```python
from build123d import *

# Parameters (mm, degrees)
SKETCH_1_R          = 13
EXTRUDE_1_DEPTH     = 5
SKETCH_2_R          = 12
CUT_EXTRUDE_1_DEPTH = 3
SKETCH_3_R          = 2.5
CUT_EXTRUDE_2_DEPTH = 2
SKETCH_4_R          = 11
FILLET_1_R          = 2
SKETCH_7_R          = 12.1
CUT_EXTRUDE_3_DEPTH = 20.05255902


with BuildPart() as part:
    # 草图1 → 凸台-拉伸1 (new body)
    with BuildSketch(Plane(origin=(0, 0, 0), x_dir=(1, 0, 0), z_dir=(0, 1, 0))):
        with Locations(Location((0, 0, 0), (0, 0, 270))):
            Circle(SKETCH_1_R)
    extrude(amount=EXTRUDE_1_DEPTH)

    # 草图2 → 切除-拉伸1 (cut)
    with BuildSketch(Plane(origin=(0, 5, 0), x_dir=(1, 0, 0), z_dir=(0, 1, 0))):
        with Locations(Location((0, 0, 0), (0, 0, 270))):
            Circle(SKETCH_2_R)
    extrude(amount=-CUT_EXTRUDE_1_DEPTH, mode=Mode.SUBTRACT)

    # 草图3 → 切除-拉伸2 (cut)
    with BuildSketch(Plane(origin=(0, 2, 0), x_dir=(1, 0, 0), z_dir=(0, 1, 0))):
        with Locations(Location((0, 0, 0), (0, 0, 270))):
            Circle(SKETCH_3_R)
    extrude(amount=-CUT_EXTRUDE_2_DEPTH, mode=Mode.SUBTRACT)

    # 草图4 → section 0 of loft_1
    with BuildSketch(Plane(origin=(0, -3, 0), x_dir=(-1, 0, 0), z_dir=(0, -1, 0)), mode=Mode.PRIVATE) as loft_1_s0:
        Circle(SKETCH_4_R)
    # loft up to a face of the part (loft_1)
    loft([loft_1_s0.sketch, Face(Wire([part.edges().sort_by_distance((-9.476592156, 0, -8.899112377))[0]]))])

    # 圆角1
    fillet_1_edges = [part.edges().sort_by_distance(p)[0] for p in [
        (11, -3, 0),
    ]]
    fillet(fillet_1_edges, radius=FILLET_1_R)

    # 草图7 → 切除-拉伸3 (cut, through all)
    with BuildSketch(Plane(origin=(0, 2, 0), x_dir=(1, 0, 0), z_dir=(0, 1, 0))):
        with Locations(Location((0, 0, 0), (0, 0, 270))):
            Circle(SKETCH_7_R)
    extrude(amount=CUT_EXTRUDE_3_DEPTH, mode=Mode.SUBTRACT)


solid = part.part
```
Model file for the job. Use its own axes, mm. A direction names the side the tool comes from. Coordinates: 2 decimals unless noted, no trailing zeros. Write each loop counter-clockwise with the first axis right and the second up, starting at its lowest first coordinate (ties: lowest second). Pieces come first, ordered by that corner, then holes. Notation, with made-up numbers: (54.5, 23.5) - (104.5, 23.5) arc R19 cw to (104.5, 49.5) - close; hole circle Ø3 at (49, -31.75). An arc over 180 degrees is marked (long way). Use a Markdown table: item, result. Add a question column.
Item 1: Band-saw the part on D-D, the plane y = 0.5. Write the cut outline in (x, z), and give its area (3 significant figures).
Item 2: Drill centre lines: line 1 along X through (y, z) = (0.65, 0); line 2 along X through (y, z) = (2.6, 0). Where is each one in solid material? Low to high.
Item 3: Drop flat-ended pins along their axis: pin 1 (3 mm diameter, centred on y = 2.5, z = 10, fed in from +X); pin 2 (8 mm diameter, centred on x = 0, z = 0, fed in from +Y); pin 3 (1.5 mm diameter, centred on x = 0.5, z = 0, fed in from +Y). Give the stop position or say it passes through.
Item 4: Band-saw the part on C-C, the plane y = -1.5. Write the cut outline in (x, z), and give its area (3 significant figures).
Item 5: Two-plate mould, pull along Z, no slides. Class faces 1 (the face through (0, -3, 0)), 2 (the face through (-7.91, 2.465, -10.316)), 3 (the face through (-2.44, 1.01, -0.54)): pulls with the +Z half, pulls with the -Z half, needs draft (parallel to the pull), parting line crosses it, or undercut.
Item 6: Band-saw the part on B-B, the plane y = 3.5. Write the cut outline in (x, z), and give its area (3 significant figures).
Item 7: 3-axis set-ups, long thin cutter, end or side, ignore diameter. For faces 4 (the face through (0, 2, 3)), 5 (the face through (-9, 5, 9)): which of +Z, -Z, +X, -X, +Y, -Y reach the whole face in a straight line?
Item 8: Band-saw the part on A-A, the plane x = 0. Write the cut outline in (y, z).
A:
| question | item | result |
|---|---|---|
| 1 | outline | circle Ø26 at (0, 0); hole circle Ø5 at (0, 0) |
| 1 | area | 511 mm² |
| 2 | line 1 | x = -13 to -2.5, 2.5 to 13 |
| 2 | line 2 | x = -13 to -12.1, 12.1 to 13 |
| 3 | pin 1 | stops at x = 9.84 |
| 3 | pin 2 | stops at y = 2 |
| 3 | pin 3 | stops at y = 0 |
| 4 | outline | circle Ø24 at (0, 0) |
| 4 | area | 452 mm² |
| 5 | face 1 | needs draft |
| 5 | face 2 | parting line crosses it |
| 5 | face 3 | undercut |
| 6 | outline | circle Ø26 at (0, 0); hole circle Ø24.2 at (0, 0) |
| 6 | area | 71.0 mm² |
| 7 | face 4 | +Y |
| 7 | face 5 | +Z, -Z, +X, -X, +Y |
| 8 | outline | (-3, -9.93) arc R2 ccw to (-2.11, -11.59) - (0, -13) - (5, -13) - (5, -12.1) - (2, -12.1) - (2, -2.5) - (0, -2.5) - (0, 2.5) - (2, 2.5) - (2, 12.1) - (5, 12.1) - (5, 13) - (0, 13) - (-2.11, 11.59) arc R2 ccw to (-3, 9.93) - close |
